Source: CAD feature listing. Evaluate the final solid. Frame: model axes, mm. Give positions to 0.01 mm unless a question says otherwise; leave off trailing zeros. Loops run counter-clockwise (first coordinate to the right, second up) from the corner with the lowest first, then second, coordinate; pieces in that order, holes last. Notation, with made-up numbers: M 48.5,27.5 L 102.5,27.5 A24 cw 102.5,44.5 Z; hole C -35.75,89 d11. An arc over 180 degrees is marked long. Put each result on its own line as item: value.
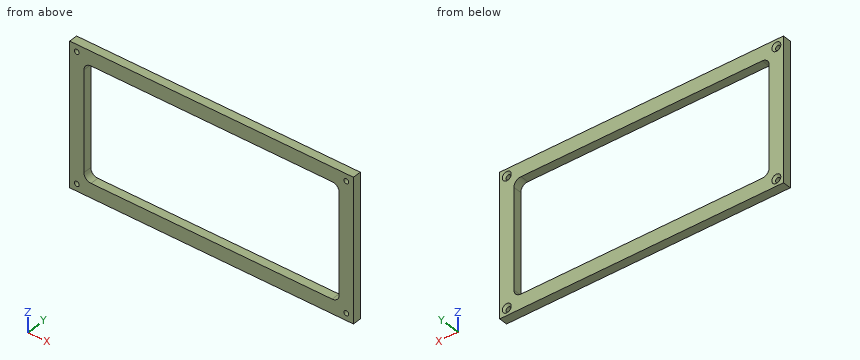
from build123d import *

# Parameters (mm, degrees)
SKETCH1_W                                           = 200
SKETCH1_H                                           = 100
BOSS_EXTRUDE1_DEPTH                                 = 6
SKETCH2_W                                           = 180
SKETCH2_H                                           = 80
CUT_EXTRUDE1_DEPTH                                  = 224.687281713
FILLET1_R                                           = 5
CSK_FOR_M3_COUNTERSUNK_FLAT_HEAD_SCREW1_D           = 3.4
CSK_FOR_M3_COUNTERSUNK_FLAT_HEAD_SCREW1_CSINK_D     = 6.3
CSK_FOR_M3_COUNTERSUNK_FLAT_HEAD_SCREW1_CSINK_ANGLE = 90


with BuildPart() as part:
    # Sketch1 → Boss-Extrude1 (new body)
    with BuildSketch(Plane(origin=(0, 0, 0), x_dir=(1, 0, 0), z_dir=(0, 1, 0))):
        with Locations((100, 50)):
            Rectangle(SKETCH1_W, SKETCH1_H)
    extrude(amount=BOSS_EXTRUDE1_DEPTH)

    # Sketch2 → Cut-Extrude1 (cut, through all)
    with BuildSketch(Plane(origin=(0, 6, 0), x_dir=(1, 0, 0), z_dir=(0, 1, 0))):
        with Locations((100, 50)):
            Rectangle(SKETCH2_W, SKETCH2_H)
    extrude(amount=-CUT_EXTRUDE1_DEPTH, mode=Mode.SUBTRACT)

    # Fillet1
    fillet1_edges = [part.edges().sort_by_distance(p)[0] for p in [
        (10, 3, -10),
        (10, 3, -90),
        (190, 3, -90),
        (190, 3, -10),
    ]]
    fillet(fillet1_edges, radius=FILLET1_R)

    # CSK for M3 Countersunk Flat Head Screw1 (through all)
    with Locations(Plane(origin=(0, 6, 0), x_dir=(1, 0, 0), z_dir=(0, 1, 0))):
        with Locations((5, 5), (5, 95), (195, 95), (195, 5)):
            CounterSinkHole(CSK_FOR_M3_COUNTERSUNK_FLAT_HEAD_SCREW1_D / 2, CSK_FOR_M3_COUNTERSUNK_FLAT_HEAD_SCREW1_CSINK_D / 2, counter_sink_angle=CSK_FOR_M3_COUNTERSUNK_FLAT_HEAD_SCREW1_CSINK_ANGLE)


solid = part.part
1. Section query B-B (x = 26.5). Output: boundary loops of the cut face in (y, z), plus the area to 3 significant figures.
Found:
outline: M 0,-100 L 6,-100 L 6,-90 L 0,-90 Z; M 0,-10 L 6,-10 L 6,0 L 0,0 Z
area: 120 mm^2
2. Section query C-C (z = -69). Output: boundary loops of the cut face in (x, y), plus the area to 3 significant figures.
Found:
outline: M 0,0 L 10,0 L 10,6 L 0,6 Z; M 190,0 L 200,0 L 200,6 L 190,6 Z
area: 120 mm^2
3. Section query A-A (y = 2.2). Output: boundary loops of the cut face in (x, z).
Found:
outline: M 0,-100 L 200,-100 L 200,0 L 0,0 Z; hole C 5,-95 d3.4; hole C 5,-5 d3.4; hole M 10,-85 A5 ccw 15,-90 L 185,-90 A5 ccw 190,-85 L 190,-15 A5 ccw 185,-10 L 15,-10 A5 ccw 10,-15 Z; hole C 195,-95 d3.4; hole C 195,-5 d3.4
4. Material intervals for line 1 (Z direction, x = 195, y = 3.3); line 2 (X direction, y = 2.95, z = -95); line 3 (Z direction, x = 116, y = 3.45), sorted ascending. Write a range as from..to.
Found:
line 1: -100..-96.7, -93.3..-6.7, -3.3..0
line 2: 0..3.3, 6.7..193.3, 196.7..200
line 3: -100..-90, -10..0
